Autodesk Inventor part; units mm, degrees
ref_plane "Work Plane2" through (0, 21, 0) normal (0, -1, 0) x (1, 0, 0)
ref_plane "Work Plane4" through (21, 0, 0) normal (-1, 0, 0) x (0, 0, 1)
ref_plane "YZ Plane" through (0, 0, 0) normal (1, 0, 0) x (0, 1, 0)
sketch "Sketch1" plane through (0, 0, 0) normal (0, 0, 1) x (1, 0, 0)
  line L0 (0, 0) -> (60, 0)
  line L1 (60, 0) -> (60, 42)
  line L2 (60, 42) -> (0, 42)
  line L3 (0, 42) -> (0, 0)
  line L4 (0, 42) -> (0, 0)
  dimension "d0" = 60
  dimension "d1" = 42
extrude "Extrusion1" add sketch "Sketch1" along normal blind 2
sketch "Sketch2" plane through (0, 0, 2) normal (0, 0, 1) x (1, 0, 0)
  circle A0 centre (21, 21) radius 11.5
  line L0 (0, 42) -> (0, 0)
  line L1 (60, 42) -> (0, 42)
  dimension "d6" = 23
  dimension "d7" = 21
  dimension "d8" = 21
extrude "Extrusion2" cut sketch "Sketch2" against normal blind 2
sketch "Sketch3" plane through (0, 0, 0) normal (0, 0, -1) x (-1, 0, 0)
  circle A0 centre (-4.95, 4.95) radius 1.25
  line L0 (0, 0) -> (-60, 0)
  line L1 (0, 42) -> (0, 0)
  dimension "d12" = 3.7
  dimension "d13" = 2.5
  dimension "d14" = 3.7
ref_plane "Work Plane2" through (0, 21, 0) normal (0, -1, 0) x (1, 0, 0)
extrude "Extrusion3" cut sketch "Sketch3" against normal through all
mirror "Mirror1" about plane through (0, 21, 0) normal (0, -1, 0) of "Extrusion3"
ref_plane "Work Plane4" through (21, 0, 0) normal (-1, 0, 0) x (0, 0, 1)
mirror "Mirror2" about plane through (21, 0, 0) normal (-1, 0, 0) of "Extrusion3", "Mirror1"
sketch "Sketch4" plane through (0, 0, 0) normal (0, 0, -1) x (-1, 0, 0)
  circle A0 centre (-21, 21) radius 11.5
  circle A1 centre (-49.8, 21) radius 2.5
  point P0 (0, 0)
  dimension "d20" = 5
  dimension "d21" = 28.8
extrude "Extrusion4" add sketch "Sketch4" along normal blind 16 contours A1
fillet "Fillet2" radius 1 1 edges at (52.3, 21, -16)
sketch "Sketch5" plane through (0, 0, 0) normal (-1, 0, 0) x (0, 0, 1)
  line L0 (0, 42) -> (0, 0)
  line L1 (0, 42) -> (2, 42)
  line L2 (0, 0) -> (2, 0)
  line L3 (2, 0) -> (2, 42)
  line L4 (2, 42) -> (0, 42)
  line L5 (0, 42) -> (0, 0)
extrude "Extrusion5" add sketch "Sketch5" along normal blind 10
sketch "Sketch6" plane through (0, 0, 0) normal (0, 0, -1) x (-1, 0, 0)
  line L0 (10, 42) -> (10, 0)
  line L1 (-60, 42) -> (10, 42)
  line L2 (10, 0) -> (3, 0)
  line L3 (3, 0) -> (3, 42)
  line L4 (3, 42) -> (10, 42)
  line L5 (10, 42) -> (10, 0)
  point P0 (0, 0)
  dimension "d32" = 7
extrude "Extrusion6" add sketch "Sketch6" along normal blind 14
sketch "Sketch7" plane through (0, 0, -14) normal (0, 0, -1) x (-1, 0, 0)
  circle A0 centre (6.5, 4) radius 2
  line L0 (3, 42) -> (3, 0)
  line L1 (3, 0) -> (10, 0)
  circle A1 centre (6.5, 21) radius 2
  circle A2 centre (6.5, 38) radius 2
  point P0 (0, 0)
  dimension "d35" = 4
  dimension "d36" = 3.5
  dimension "d37" = 4
  dimension "d40" = 17
extrude "Extrusion7" add sketch "Sketch7" along normal blind 2
chamfer "Chamfer2" distance 1 angle 45 2 edges at (35.8, 4.95, 0) (35.8, 37.05, 0)
sketch "Sketch9" plane through (0, 0, 0) normal (0, 0, -1) x (-1, 0, 0)
  circle A0 centre (-4.95, 4.95) radius 1.25
  circle A1 centre (-4.95, 37.05) radius 1.25
  circle A2 centre (-4.95, 4.95) radius 2.5
  circle A3 centre (-4.95, 37.05) radius 2.5
  point P0 (0, 0)
  dimension "d50" = 5
  dimension "d51" = 5
extrude "Extrusion8" add sketch "Sketch9" along normal blind 2
fillet "Fillet3" radius 2 2 edges at (7.45, 4.95, 0) (7.45, 37.05, 0)
properties part number "MotorKuggHolder"
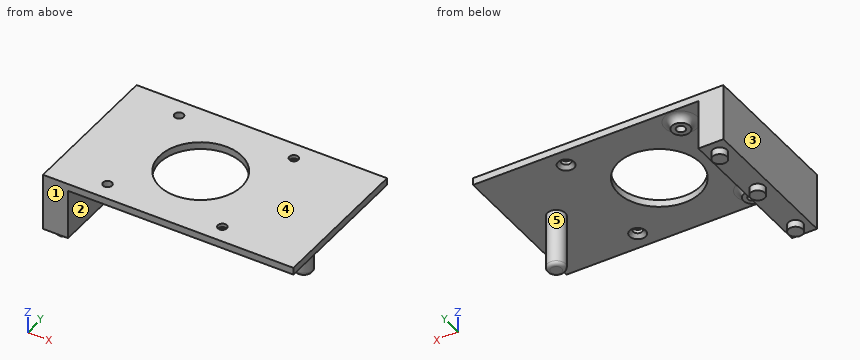
CAD build for the part. Positions are in the model's coordinates, mm. Face numbers are marked on the shaded views. A direction names the side the tool comes from. Coordinates: 2 decimals unless noted, no trailing zeros. Loops run counter-clockwise (first coordinate to the right, second up) from the corner with the lowest first, then second, coordinate; pieces in that order, holes last. Notation, with made-up numbers: (51.25, -17) - (83.25, -17) arc R10 cw to (83.25, -2) - close; hole circle Ø9 at (35.5, 17). An arc over 180 degrees is marked (long way). Write item = value, one per line. Start each with the question number.
Q1. Cut at B-B, the plane z = -7.5. List the corners of the cut face in (x, y), then the cut area to 3 significant figures.
Q2. Cut at C-C, the plane x = 21. List the corners of the cut face in (y, z).
Q3. Cut at D-D, the plane z = -1.25. List the corners of the cut face in (x, y), then the cut area to 3 significant figures.
Q4. Drill centre lines: L1, parallel to Y at x = 37.05, z = 1.5; L2, parallel to X at y = 6, z = 1.25; L3, parallel to Z at x = 47, y = 9.5. Where is each one in solid material? Low to high.
Q5. Cut at A-A, the plane x = 4.95. Give the number of separate pieces and of enclosed holes in the cut face, then the cut area to 3 significant figures.
Q6. Flat gauge pins, fed straight in: pin 1 Ø5.5 at (x, y) = (5.5, 6) entering from -Z; pin 2 Ø4 at (x, y) = (37.05, 37.05) entering from -Z; pin 3 Ø4 at (y, z) = (28, -10.5) entering from +X. Where does each tip first touch, or does it go through?
Q7. Which spindle directions (+Z, -Z, +X, -X, +Y, -Y) get a long thin tool onto all of the face, cutting with end or side? Do the marked faces 4 and 5. Say none if no direction does.
Q8. Pull direction X, two halves, no side cores. Call the marked faces 1, 2 and 3: pulls with the +X half, pulls with the -X half, needs draft (parallel to the pull), parting line crosses it, or undercut.
Computed:
q1.outline = (-10, 0) - (-3, 0) - (-3, 42) - (-10, 42) - close; circle Ø5 at (49.8, 21)
q1.area = 314 mm²
q2.outline = (0, 0) - (9.5, 0) - (9.5, 2) - (0, 2) - close; (32.5, 0) - (42, 0) - (42, 2) - (32.5, 2) - close
q3.outline = (-10, 0) - (-3, 0) - (-3, 42) - (-10, 42) - close; circle Ø5.29 at (4.95, 4.95); circle Ø5.29 at (4.95, 37.05); circle Ø5 at (49.8, 21); hole circle Ø2.5 at (4.95, 4.95); hole circle Ø2.5 at (4.95, 37.05)
q3.area = 348 mm²
q4.L1 = 0 to 3.7, 6.2 to 35.8, 38.3 to 42
q4.L2 = -10 to 4.27, 5.63 to 36.37, 37.73 to 60
q4.L3 = 0 to 2
q5.separate_pieces = 3
q5.enclosed_holes = 0
q5.area = 87.4 mm²
q6.pin_1 = -2
q6.pin_2 = 0.25
q6.pin_3 = -3
q7.face_4 = +Z, +X, -X, +Y, -Y
q7.face_5 = -Z
q8.face_1 = needs draft
q8.face_2 = undercut
q8.face_3 = pulls with the -X half
